```python
from build123d import *

# Parameters (mm, degrees)
SKETCH1_R               = 12.7
BOSS_EXTRUDE1_DEPTH     = 13.16
CUT_EXTRUDE4_DEPTH      = 13.7
CUT_EXTRUDE4_DEPTH_BACK = 13.7
SKETCH4_R               = 1.595
CUT_EXTRUDE9_DEPTH      = 4.32


with BuildPart() as part:
    # Sketch1 → Boss-Extrude1 (new body)
    with BuildSketch(Plane(origin=(0, 0, 0), x_dir=(1, 0, 0), z_dir=(0, 1, 0))):
        Circle(SKETCH1_R)
    extrude(amount=BOSS_EXTRUDE1_DEPTH)

    # Sketch2 → Cut-Extrude4 (cut, two sides)
    with BuildSketch(Plane.XY) as cut_extrude4_sk:
        Polygon((-77.620622605, 30.565883462), (-12.7, 13.16), (12.7, 6.35), (77.620622605, -11.055883462), (112.43238953, 118.785361749), (-42.808855681, 160.407128673), align=None)
    extrude(amount=CUT_EXTRUDE4_DEPTH, mode=Mode.SUBTRACT)
    extrude(cut_extrude4_sk.sketch, amount=-CUT_EXTRUDE4_DEPTH_BACK, mode=Mode.SUBTRACT)

    # Sketch4 → Cut-Extrude9 (cut)
    with BuildSketch(Plane(origin=(0, 0, 0), x_dir=(1, 0, 0), z_dir=(0, 1, 0))):
        with Locations((-9.525, 0)):
            Circle(SKETCH4_R)
        with Locations((0.005, 0)):
            Circle(SKETCH4_R)
        with Locations((9.535, 0)):
            Circle(SKETCH4_R)
        with Locations((4.7625, 8.248891971)):
            Circle(SKETCH4_R)
        with Locations((4.7625, -8.248891971)):
            Circle(SKETCH4_R)
    extrude(amount=CUT_EXTRUDE9_DEPTH, mode=Mode.SUBTRACT)


solid = part.part
```
The listing builds one solid part. Answer for the finished solid, in the listing's coordinates (mm). A direction names the side the tool comes from. Give positions to 0.01 mm unless a question says otherwise; leave off trailing zeros. Loops run counter-clockwise (first coordinate to the right, second up) from the corner with the lowest first, then second, coordinate; pieces in that order, holes last. Notation, with made-up numbers: (-38.75, -18) - (-20.75, -18) arc R20 cw to (-20.75, 18) - close; hole circle Ø9 at (55, -11.5). An arc over 180 degrees is marked (long way). Answer as CSV lines item,"result". Start each with the question number.
Item 1: A cutting plane is placed at B-B on x = -9.25. Determine the outline of the cut face in (y, z), then the cut area to 3 significant figures.
Item 2: Each of these flat-tipped pins is pushed along its axis until it touches: pin 1 (4 mm diameter, centred on y = 5, z = 6, fed in from -X); pin 2 (3.5 mm diameter, centred on x = -9.525, z = 0, fed in from +Y); pin 3 (1.6 mm diameter, centred on x = 9, z = -0.5, fed in from -Y). Where does it stop, or does it pass through?
Item 3: Find the intervals of material crossed by line 1 (X direction, y = 2.55, z = 0); line 2 (X direction, y = 2.5, z = -0.75); line 3 (Z direction, x = -10.75, y = 2.75), in increasing order. Write a range as from..to.
Item 4: For faces 1 (the face through (-0.178, 9.803, -0.178)), 2 (the face through (3.59, 2.13, 7.17)), determine the directions among +Z, -Z, +X, -X, +Y, -Y from which every point of the face is accessible in a straight line to the end or side of a thin tool.
Item 5: A cutting plane is placed at C-C on x = 0. Determine the outline of the cut face in (y, z) (3 decimals), then the cut area to 3 significant figures.
Item 6: A cutting plane is placed at A-A on z = 0. Determine the outline of the cut face in (x, y).
Item 7: The mould has two halves that part along X. Classify faces 3 (the face through (-12.688, 5.026, -0.558)), 4 (the face through (0, 4.32, 0)), 5 (the face through (0, 0, 3)): +X half, -X half, draft (parallel to the pull), parting line (faces both ways), or undercut.
Item 8: A cutting plane is placed at D-D on y = 9.5. Determine the outline of the cut face in (x, z), then the cut area to 3 significant figures.
Found:
1,outline,"(0, -8.7) - (12.24, -8.7) - (12.24, 8.7) - (0, 8.7) - (0, 1.57) - (4.32, 1.57) - (4.32, -1.57) - (0, -1.57) - close"
1,area,"199 mm^2"
2,pin 1,"stops at x = -12.05"
2,pin 2,"stops at y = 12.78"
2,pin 3,"stops at y = 4.32"
3,line 1,"x = -12.7..-11.12, -7.93..-1.59, 1.6..7.94, 11.13..12.7"
3,line 2,"x = -12.68..-10.93, -8.12..-1.4, 1.41..8.13, 10.94..12.68"
3,line 3,"z = -6.76..-1.02, 1.02..6.76"
4,face 1,"+Z, -Z, +X, +Y"
4,face 2,"-Y"
5,outline,"(0, -12.7) - (9.755, -12.7) - (9.755, 12.7) - (0, 12.7) - (0, 1.595) - (4.32, 1.595) - (4.32, -1.595) - (0, -1.595) - close"
5,area,"234 mm^2"
6,outline,"(-12.7, 0) - (-11.12, 0) - (-11.12, 4.32) - (-7.93, 4.32) - (-7.93, 0) - (-1.59, 0) - (-1.59, 4.32) - (1.6, 4.32) - (1.6, 0) - (7.94, 0) - (7.94, 4.32) - (11.13, 4.32) - (11.13, 0) - (12.7, 0) - (12.7, 6.35) - (-12.7, 13.16) - close"
7,face 3,"parting line"
7,face 4,"undercut"
7,face 5,"draft"
8,outline,"(0.95, -12.66) - (0.95, 12.66) arc R12.7 ccw (long way) to start"
8,area,"277 mm^2"
